Design review of the part built by this model. Coordinates are the model's own, in mm. Face numbers are marked on the shaded views. Give positions to 0.01 mm unless a question says otherwise; leave off trailing zeros. Write each loop counter-clockwise with the first axis right and the second up, starting at its lowest first coordinate (ties: lowest second). Pieces come first, ordered by that corner, then holes.
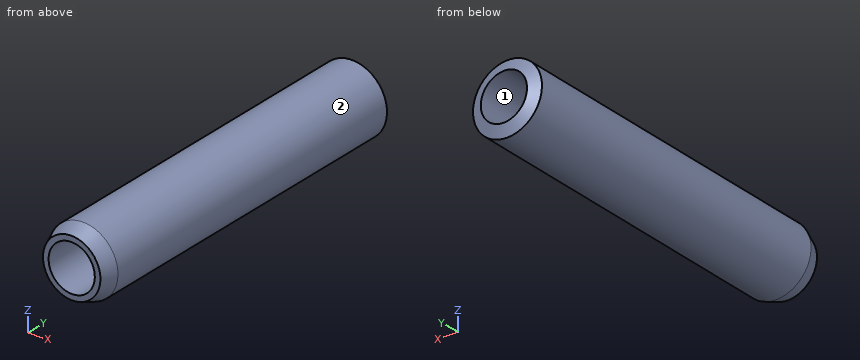
```python
from build123d import *

# Parameters (mm, degrees)
SKETCH1_R           = 20
BOSS_EXTRUDE1_DEPTH = 207.198025
SKETCH2_R           = 13.399724126
CUT_EXTRUDE1_DEPTH  = 210.119634573
CHAMFER1_SIZE       = 3.349594
CHAMFER1_SIZE_2     = 8.537032


with BuildPart() as part:
    # Sketch1 → Boss-Extrude1 (new body)
    with BuildSketch(Plane(origin=(0, 0, 0), x_dir=(1, 0, 0), z_dir=(0, 1, 0))):
        with Locations(Location((0, 0, 0), (0, 0, 90))):
            Circle(SKETCH1_R)
    extrude(amount=BOSS_EXTRUDE1_DEPTH)

    # Sketch2 → Cut-Extrude1 (cut, through all)
    with BuildSketch(Plane(origin=(0, 0, 0), x_dir=(1, 0, 0), z_dir=(0, 1, 0))):
        with Locations(Location((0, 0, 0), (0, 0, 90))):
            Circle(SKETCH2_R)
    extrude(amount=CUT_EXTRUDE1_DEPTH, mode=Mode.SUBTRACT)

    # Chamfer1
    # the kernel refuses this chamfer: 8.537032, 3.349594 mm, written as the material it takes off along each edge
    with BuildSketch(Plane(origin=(0, 207.198025, 0), x_dir=(0, 0, -1), z_dir=(1, 0, 0))) as chamfer1_piece_1:
        Polygon((20, -CHAMFER1_SIZE), (20 - CHAMFER1_SIZE_2, 0), (20, 0), align=None)
    revolve(axis=Axis((0, 207.198025, 0), (0, 1, 0)), mode=Mode.SUBTRACT)
    with BuildSketch(Plane(origin=(0, 0, 0), x_dir=(0, 0, -1), z_dir=(1, 0, 0))) as chamfer1_piece_2:
        Polygon((20, CHAMFER1_SIZE_2), (20 - CHAMFER1_SIZE, 0), (20, 0), align=None)
    revolve(axis=Axis((0, 0, 0), (0, 1, 0)), mode=Mode.SUBTRACT)


solid = part.part
```
(1) Mouldability with a two-part tool opening along Z and no side actions: class the marked faces 1 and 2 as pulls with the +Z half, pulls with the -Z half, needs draft (parallel to the pull), parting line crosses it, or undercut.
Resolved:
face 1: undercut
face 2: parting line crosses it
(2) Clearance check with flat-ended pins moving along their axes: P1, Ø2, axis at x = 13.5, z = 6.5, coming from the -Y side; P2, Ø5, axis at y = 107, z = -11, coming from the +X side; P3, Ø6, axis at y = 29, z = 3, coming from the +X side; P4, Ø4, axis at x = 12, y = 115.5, coming from the -Z side. State where each tip first meets the part, or that it passes through.
Resolved:
P1: stops at y = 0
P2: stops at x = 18.1
P3: stops at x = 20
P4: stops at z = -17.32
(3) Consider section C-C, the plane y = 174.5. Give the boundary of the cut face in (x, z), then the cut area to 3 significant figures.
Resolved:
outline: circle Ø40 at (0, 0); hole circle Ø26.8 at (0, 0)
area: 693 mm2
(4) Consider section A-A, the plane z = 0. Give the boundary of the cut face in (x, y), then the cut area to 3 significant figures.
Resolved:
outline: (-20, 8.54) - (-16.65, 0) - (-13.4, 0) - (-13.4, 206.44) - (-20, 203.85) - close; (13.4, 0) - (16.65, 0) - (20, 8.54) - (20, 203.85) - (13.4, 206.44) - close
area: 2,680 mm2
(5) To check wall thickness, follow L1, parallel to X at y = 53, z = 0; L2, parallel to X at y = 196, z = -8; L3, parallel to Z at x = -3, y = 188.5. State the ranges of each line that lie inside material, in increasing order.
Resolved:
L1: x = -20 to -13.4, 13.4 to 20
L2: x = -18.33 to -10.75, 10.75 to 18.33
L3: z = -19.77 to -13.06, 13.06 to 19.77
(6) Consider section B-B, the plane x = 0. Give the boundary of the cut face in (y, z), then the cut area to 3 significant figures.
Resolved:
outline: (0, -16.65) - (8.54, -20) - (203.85, -20) - (206.44, -13.4) - (0, -13.4) - close; (0, 13.4) - (206.44, 13.4) - (203.85, 20) - (8.54, 20) - (0, 16.65) - close
area: 2,680 mm2
